Geometry: final body of the model. Coordinates: model frame, mm. Face numbers are marked on the shaded views. A direction names the side the tool comes from. Round coordinates to 2 decimals unless told otherwise and drop trailing zeros. Order: outer loops, then holes, each group sorted by start corner. A loop starts at its lowest first (then second) coordinate and runs counter-clockwise, first axis right, second up. Notation, with made-up numbers: M -22,-31.75 L -4,-31.75 A21 cw -4,-5.75 Z; hole C 20.25,53.25 d8. An arc over 180 degrees is marked long. Return JSON: item names as keys, results as strings. Group by question number.
Q1. Ray query, probe 1 along X at (y, z) = (0, 16) (3 decimals); probe 2 along Y at (x, z) = (0, 23) (3 decimals); probe 3 along X at (y, z) = (-1.5, 19) (3 decimals). Return the intervals inside material, ascending.
Q2. Access query for the marked faces 1, 2, 3, 4 and 5. Directions: +Z, -Z, +X, -X, +Y, -Y. A direction counts if a zero-diameter tool reaches every point of the face in a straight line with its end or side. Return the directions, or none.
Q3. Contact query for flat-ended pins moving along their axis: pin 1 (10 mm diameter, centred on x = -2, y = 19.5, fed in from +Z); pin 2 (11.5 mm diameter, centred on x = 0, y = -3, fed in from +Z); pin 3 (5 mm diameter, centred on x = -35.5, z = 5.5, fed in from -Y). Output: stop coordinate, or through.
Q4. Cut plane B-B on x = -53.5. Output: boundary loops of the cut face in (y, z), and give its area (3 significant figures).
Q5. Mould query, pull axis X, two halves, no side actions, for the marked faces 6, 7, 8 and 9. Classes: released by +X, released by -X, zero draft, split by the parting line, or undercut.
Q6. Cut plane C-C on y = -30. Output: boundary loops of the cut face in (x, z) (3 decimals), and give its area (3 significant figures).
Q7. Cut plane A-A on z = 17. Output: boundary loops of the cut face in (x, y) (3 decimals).
Q8. Cut plane D-D on z = -14.5. Output: boundary loops of the cut face in (x, y) (3 decimals), and give its area (3 significant figures).
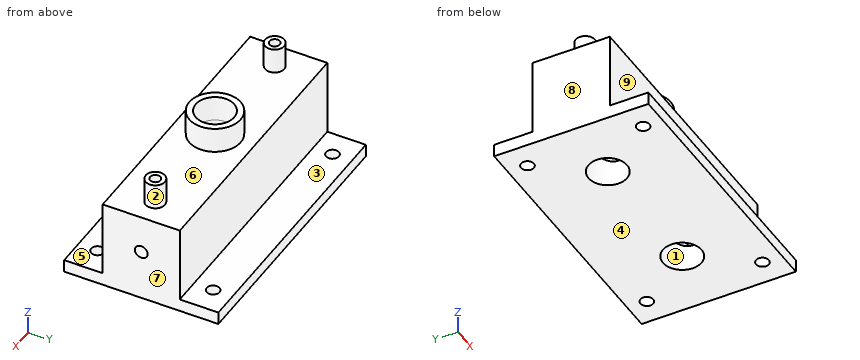
```python
from build123d import *

# Parameters (mm, degrees)
F0_W      = 38.1
F0_H      = 38.1
F1_DEPTH  = 66.675
F3_R      = 12.7
F4_DEPTH  = 120.65
F5_W      = 133.35
F5_H      = 76.2
F5_R      = 3.175
F6_DEPTH  = 6.35
F7_R      = 9.525
F8_DEPTH  = 25.4
F9_R      = 9.525
F9_R_2    = 3.175
F10_DEPTH = 19.05
F11_R     = 4.7625
F11_R_2   = 2.5527
F11_R_3   = 12.7
F11_R_4   = 9.525
F12_DEPTH = 12.7
F13_R     = 3.175
F14_DEPTH = 12.7


with BuildPart() as f1:
    # F0 (on Right) → F1 (new body, symmetric)
    with BuildSketch(Plane.YZ):
        Rectangle(F0_W, F0_H)
    extrude(amount=F1_DEPTH, both=True)

    # F3 (on offset) → F4 (cut)
    with BuildSketch(Plane.YZ.offset(60.325)):
        Circle(F3_R)
    extrude(amount=-F4_DEPTH, mode=Mode.SUBTRACT)

    # F5 (on face) → F6 (join)
    with BuildSketch(Plane(origin=(0, 0, -19.05), x_dir=(1, 0, 0), z_dir=(0, 0, -1))):
        Rectangle(F5_W, F5_H)
        with Locations((-53.975, -28.575)):
            Circle(F5_R, mode=Mode.SUBTRACT)
        with Locations((53.975, -28.575)):
            Circle(F5_R, mode=Mode.SUBTRACT)
        with Locations((-53.975, 28.5496)):
            Circle(F5_R, mode=Mode.SUBTRACT)
        with Locations((53.975, 28.5496)):
            Circle(F5_R, mode=Mode.SUBTRACT)
    extrude(amount=F6_DEPTH)

    # F7 (on face) → F8 (cut)
    with BuildSketch(Plane(origin=(0, 0, -25.4), x_dir=(1, 0, 0), z_dir=(0, 0, -1))):
        with Locations((-33.655, 0)):
            Circle(F7_R)
        with Locations((33.655, 0)):
            Circle(F7_R)
    extrude(amount=-F8_DEPTH, mode=Mode.SUBTRACT)

    # F9 (on face) → F10 (cut)
    with BuildSketch(Plane.XY.offset(19.05)):
        Circle(F9_R)
        with Locations((-53.975, 0)):
            Circle(F9_R_2)
        with Locations((53.975, 0)):
            Circle(F9_R_2)
    extrude(amount=-F10_DEPTH, mode=Mode.SUBTRACT)

    # F11 (on face) → F12 (join)
    with BuildSketch(Plane.XY.offset(19.05)):
        with Locations((-53.975, 0)):
            Circle(F11_R)
        with Locations((-53.975, 0)):
            Circle(F11_R_2, mode=Mode.SUBTRACT)
        Circle(F11_R_3)
        Circle(F11_R_4, mode=Mode.SUBTRACT)
        with Locations((53.975, 0)):
            Circle(F11_R)
        with Locations((53.975, 0)):
            Circle(F11_R_2, mode=Mode.SUBTRACT)
    extrude(amount=F12_DEPTH)

    # F13 (on face) → F14 (cut)
    with BuildSketch(Plane.YZ.offset(66.675)):
        Circle(F13_R)
    extrude(amount=-F14_DEPTH, mode=Mode.SUBTRACT)


solid = f1.part
```
Result sheet:
{
 "1": {"probe 1": "x = -66.675 to -57.15, -50.8 to -9.525, 9.525 to 50.8, 57.15 to 66.675", "probe 2": "y = -12.7 to -9.525, 9.525 to 12.7", "probe 3": "x = -66.675 to -56.773, -51.177 to -9.406, 9.406 to 51.177, 56.773 to 66.675"},
 "2": {"face 1": "-Z", "face 2": "+Z", "face 3": "+Z, +X, -X, +Y", "face 4": "-Z, +X, -X, +Y, -Y", "face 5": "+Z, +X, -X, -Y"},
 "3": {"pin 1": "stops at z = 19.05", "pin 2": "stops at z = -9.2", "pin 3": "stops at y = -19.05"},
 "4": {"outline": "M -38.1,-25.4 L -31.69,-25.4 L -31.69,-19.05 L -38.1,-19.05 Z; M -25.41,-25.4 L 25.44,-25.4 L 25.44,-19.05 L 19.05,-19.05 L 19.05,19.05 L 4.74,19.05 L 4.74,31.75 L 2.51,31.75 L 2.51,19.05 L 3.14,19.05 L 3.14,12.31 A12.7 cw long -3.14,12.31 L -3.14,19.05 L -2.51,19.05 L -2.51,31.75 L -4.74,31.75 L -4.74,19.05 L -19.05,19.05 L -19.05,-19.05 L -25.41,-19.05 Z; M 31.71,-25.4 L 38.1,-25.4 L 38.1,-19.05 L 31.71,-19.05 Z", "area": "1,370 mm²"},
 "5": {"face 6": "undercut", "face 7": "released by +X", "face 8": "released by -X", "face 9": "zero draft"},
 "6": {"outline": "M -66.675,-25.4 L -56.799,-25.4 L -56.799,-19.05 L -66.675,-19.05 Z; M -51.151,-25.4 L 51.151,-25.4 L 51.151,-19.05 L -51.151,-19.05 Z; M 56.799,-25.4 L 66.675,-25.4 L 66.675,-19.05 L 56.799,-19.05 Z", "area": "775 mm²"},
 "7": {"outline": "M -66.675,-19.05 L 66.675,-19.05 L 66.675,19.05 L -66.675,19.05 Z; hole C -53.975,0 d6.35; hole C 0,0 d19.05; hole C 53.975,0 d6.35"},
 "8": {"outline": "M -66.675,-19.05 L 66.675,-19.05 L 66.675,19.05 L -66.675,19.05 Z; hole C -33.655,0 d19.05; hole C 33.655,0 d19.05", "area": "4,510 mm²"}
}
